Could you check a few things on this model? Use its own coordinates, in mm. A direction names the side the tool comes from. Give positions to 0.01 mm unless a question says otherwise; leave off trailing zeros. Order: outer loops, then holes, each group sorted by start corner. A loop starts at its lowest first (then second) coordinate and runs counter-clockwise, first axis right, second up. Notation, with made-up numbers: (38.5, 28.5) -> (83.5, 28.5) arc R34 ccw to (83.5, 65.5) -> close; hole circle Ø6 at (70, 76.5). An arc over 180 degrees is marked (long way). One line per item, written item: value.
```python
from build123d import *

# Parameters (mm, degrees)
F1_DEPTH = 2.54
F3_DEPTH = 127


# Not quite as in the source:
# - ends of sketch curves that miss each other by under 0.0002 mm in the source are joined


with BuildPart() as f1:
    # F0 (on Top) → F1 (new body)
    with BuildSketch(Plane.XY):
        Polygon((34.9249995572, 23.8301315939), (3.1749995572, 42.1610026407), (0, 43.994091056), (-38.1000004709, 21.997045528), (-38.1000004709, -21.997045528), (0, -43.994091056), (38.1000004709, -21.997045528), (38.1000004709, 21.997045528), align=None)
        Polygon((0, 36.6617420935), (31.75, 18.3308710468), (31.75, -18.3308710468), (0, -36.6617420935), (-31.75, -18.3308710468), (-31.75, 18.3308710468), align=None, mode=Mode.SUBTRACT)
    extrude(amount=F1_DEPTH)

    # F2 (on face) → F3 (join)
    with BuildSketch(Plane.XY.offset(2.54)):
        with BuildLine():
            ThreePointArc((-38.1000004709, 19.3844549358), (-35.2889631462, 16.6640411269), (-31.75, 18.3308710468))
            ThreePointArc((-31.75, 18.3308710468), (-31.403147802, 19.1639531761), (-31.2848175618, 20.0585649554))
            ThreePointArc((-31.2848175618, 20.0585649554), (-32.7035344951, 22.8425648101), (-35.7897937807, 23.3308439825))
            Line((-35.7897937807, 23.3308439825), (-37.0276020707, 22.616195033))
            ThreePointArc((-37.0276020707, 22.616195033), (-37.7159751418, 21.7610765108), (-38.1000004709, 20.7326749751))
            Line((-38.1000004709, 20.7326749751), (-38.1000004709, 19.3844549358))
        make_face()
        with BuildLine():
            ThreePointArc((35.8374259749, 23.3033424061), (32.0759629522, 22.2291160887), (31.75, 18.3308710468))
            ThreePointArc((31.75, 18.3308710468), (35.2686397989, 16.6449401257), (38.1000004709, 19.329448619))
            Line((38.1000004709, 19.329448619), (38.1000004709, 20.758746518))
            ThreePointArc((38.1000004709, 20.758746518), (37.7036332461, 21.7824533156), (37.0050252462, 22.6292292285))
            Line((37.0050252462, 22.6292292285), (35.8374259749, 23.3033424061))
        make_face()
        with BuildLine():
            ThreePointArc((3.4325778187, -40.1026625239), (2.4277039418, -37.6725121227), (0, -36.6617420935))
            ThreePointArc((0, -36.6617420935), (-3.2193789061, -38.8660080857), (-2.3102066902, -42.6602926015))
            Line((-2.3102066902, -42.6602926015), (-1.0723984002, -43.374941551))
            ThreePointArc((-1.0723984002, -43.374941551), (0.0123424988, -43.5435308567), (1.0949770186, -43.3619057795))
            Line((1.0949770186, -43.3619057795), (2.2625698225, -42.6877957599))
            ThreePointArc((2.2625698225, -42.6877957599), (3.1264590528, -41.5214500837), (3.4325778187, -40.1026625239))
        make_face()
    extrude(amount=F3_DEPTH)


solid = f1.part
```
1) Suppose I cut it at C-C, the plane x = 20.5. Write out the boundary of the cut face in (y, z).
Answer below:
outline: (-32.16, 0) -> (-24.83, 0) -> (-24.83, 2.54) -> (-32.16, 2.54) -> close; (24.83, 0) -> (32.16, 0) -> (32.16, 2.54) -> (24.83, 2.54) -> close
2) Suppose I cut it at D-D, the plane y = 38.5. Write out the boundary of the cut face in (x, z), then the cut area to 3 significant figures.
Answer below:
outline: (-9.52, 0) -> (9.52, 0) -> (9.52, 2.54) -> (-9.52, 2.54) -> close
area: 48.3 mm2
3) Suppose I cut it at B-B, the plane z = 38.5. Write out the boundary of the cut face in (x, y), then the cut area to 3 significant figures.
Answer below:
outline: (-38.1, 19.38) arc R3.44 ccw (long way) to (-35.79, 23.33) -> (-37.03, 22.62) arc R3.44 ccw to (-38.1, 20.73) -> close; (-2.31, -42.66) -> (-1.07, -43.37) arc R3.44 ccw to (1.09, -43.36) -> (2.26, -42.69) arc R3.44 ccw (long way) to start; (35.84, 23.3) arc R3.44 ccw (long way) to (38.1, 19.33) -> (38.1, 20.76) arc R3.44 ccw to (37.01, 22.63) -> close
area: 111 mm2
4) For faces 3 (the flat face through (35, 20, 129.54)), 4 (the flat face through (-16.097, 27.368, 1.252)), which set-ups out of +Z, -Z, +X, -X, +Y, -Y let a thin tool reach every point of the face, with its end or its side?
Answer below:
face 3: +Z, +X, -X, +Y, -Y
face 4: +Z, -Z
5) If I drill on line 1 along Z through (x, y) = (5.5, -40); line 2 along Y through (x, z) = (0, 73.5); line 3 along Y through (x, z) = (32, 21), over which ranges is the centre line in solid material (lowest first)?
Answer below:
line 1: z = 0 to 2.54
line 2: y = -43.54 to -36.66
line 3: y = 17.95 to 22.13
6) For P1, Ø20.5, axis at x = 16, y = 37, coming from the +Z side; P2, Ø6, axis at x = 5.5, z = 52, coming from the +Y side; P3, Ø4, axis at x = 30, z = 98, coming from the +Y side, each with a flat end and sliding along its axis, tell me the tip position at first contact or that it passes through.
Answer below:
P1: stops at z = 2.54
P2: stops at y = -37.75
P3: stops at y = 22.13
7) Suppose I cut it at A-A, the plane y = -4. Write out the boundary of the cut face in (x, z).
Answer below:
outline: (-38.1, 0) -> (-31.75, 0) -> (-31.75, 2.54) -> (-38.1, 2.54) -> close; (31.75, 0) -> (38.1, 0) -> (38.1, 2.54) -> (31.75, 2.54) -> close
8) We'd pull the mould along Y, two halves only. Please class faces 1 (the flat face through (0, -40, 129.54)), 2 (the flat face through (15.653, 27.625, 1.252)): +Y half, -Y half, draft (parallel to the pull), parting line (faces both ways), or undercut.
Answer below:
face 1: draft
face 2: undercut
